```python
from build123d import *

# Parameters (mm, degrees)
PAD_DEPTH            = 10
SKETCH001_R          = 2.5
POCKET_DEPTH         = 19.79999
SKETCH002_R          = 2.125
POCKET001_DEPTH      = 28.143136
SKETCH003_R          = 4
SKETCH003_R_2        = 2.125
PAD001_DEPTH         = 5
SKETCH004_R          = 2.125
SKETCH004_R_2        = 1.5
PAD002_DEPTH         = 2
SKETCH005_W          = 20
SKETCH005_H          = 5
SKETCH005_W_2        = 9.142136
SKETCH005_H_2        = 1
POCKET002_DEPTH      = 28.143136
POCKET002_DEPTH_BACK = -10.001
SKETCH006_R          = 1.6
POCKET003_DEPTH      = 15.001
POCKET004_DEPTH      = 3
SKETCH008_R          = 5
POCKET005_DEPTH      = 2


with BuildPart() as part:
    # Sketch → Pad (new body, symmetric)
    with BuildSketch(Plane.XZ):
        Polygon((0, 0), (0, 20), (-14.142136, 34.142136), (-19.79899, 28.485281), (-8, 16.686292), (-8, 0), align=None)
    extrude(amount=PAD_DEPTH, both=True)

    # Sketch001 (on Face1 of Pad) → Pocket (cut, through all)
    with BuildSketch(Plane(origin=(0, 0, 0), x_dir=(0, 0, 1), z_dir=(1, 0, 0))):
        with Locations((10, 0)):
            Circle(SKETCH001_R)
    extrude(amount=-POCKET_DEPTH, mode=Mode.SUBTRACT)

    # Sketch002 (on Face5 of Pocket) → Pocket001 (cut, through all)
    with BuildSketch(Plane(origin=(10, 0, 10), x_dir=(-0.707107, 0, 0.707107), z_dir=(0.707107, 0, 0.707107))):
        with Locations((24.142136, 0)):
            Circle(SKETCH002_R)
    extrude(amount=-POCKET001_DEPTH, mode=Mode.SUBTRACT)

    # Sketch003 (on Face5 of Pocket001) → Pad001 (join)
    with BuildSketch(Plane(origin=(10, 0, 10), x_dir=(-0.707107, 0, 0.707107), z_dir=(0.707107, 0, 0.707107))):
        with Locations((24.142136, 0)):
            Circle(SKETCH003_R)
        with Locations((24.142136, 0)):
            Circle(SKETCH003_R_2, mode=Mode.SUBTRACT)
    extrude(amount=PAD001_DEPTH)

    # Sketch004 (on Face11 of Pad001) → Pad002 (join)
    with BuildSketch(Plane(origin=(13.535534, 0, 13.535534), x_dir=(-0.707107, 0, 0.707107), z_dir=(0.707107, 0, 0.707107))):
        with Locations((24.142136, 0)):
            Circle(SKETCH004_R)
        with Locations((24.142136, 0)):
            Circle(SKETCH004_R_2, mode=Mode.SUBTRACT)
    extrude(amount=-PAD002_DEPTH)

    # Sketch005 (on Face5 of Pad002) → Pocket002 (cut, two sides)
    with BuildSketch(Plane(origin=(10, 0, 10), x_dir=(-0.707107, 0, 0.707107), z_dir=(0.707107, 0, 0.707107))) as pocket002_sk:
        with Locations((24.142136, 7.5)):
            Rectangle(SKETCH005_W, SKETCH005_H)
        with Locations((24.142136, -7.5)):
            Rectangle(SKETCH005_W, SKETCH005_H)
        with Locations((29.571068, 0)):
            Rectangle(SKETCH005_W_2, SKETCH005_H_2)
    extrude(amount=-POCKET002_DEPTH, mode=Mode.SUBTRACT)
    extrude(pocket002_sk.sketch, amount=-POCKET002_DEPTH_BACK, mode=Mode.SUBTRACT)

    # Sketch006 (on Face16 of Pocket002) → Pocket003 (cut, through all)
    with BuildSketch(Plane.XZ.offset(5)):
        with Locations((-14.142136, 28.485281)):
            Circle(SKETCH006_R)
    extrude(amount=-POCKET003_DEPTH, mode=Mode.SUBTRACT)

    # Sketch007 (on Face10 of Pocket003) → Pocket004 (cut)
    with BuildSketch(Plane(origin=(0, 5, 0), x_dir=(1, 0, 0), z_dir=(0, 1, 0))):
        Polygon((-11.002877, -29.326443), (-11.844039, -26.187184), (-14.983298, -25.346022), (-17.281395, -27.644119), (-16.440233, -30.783378), (-13.300974, -31.62454), align=None)
    extrude(amount=-POCKET004_DEPTH, mode=Mode.SUBTRACT)

    # Sketch008 (on Face9 of Pocket004) → Pocket005 (cut)
    with BuildSketch(Plane(origin=(-8, 0, 0), x_dir=(0, 0, -1), z_dir=(-1, 0, 0))):
        with Locations((-10, 0)):
            Circle(SKETCH008_R)
    extrude(amount=-POCKET005_DEPTH, mode=Mode.SUBTRACT)


solid = part.part
```
Geometry: final body of the model. Coordinates: model frame, mm. A direction names the side the tool comes from. Coordinates: 2 decimals unless noted, no trailing zeros. Order: outer loops, then holes, each group sorted by start corner. A loop starts at its lowest first (then second) coordinate and runs counter-clockwise, first axis right, second up. Notation, with made-up numbers: (74, 62.25) -> (96, 62.25) arc R24 ccw to (96, 81.25) -> close; hole circle Ø5 at (9.5, -5.5). An arc over 180 degrees is marked (long way). Write each question's results on one line, items separated by ' | '. Start each with the question number.
1) Material intervals for line 1 along Y through (x, z) = (-6.75, 10); line 2 along Z through (x, y) = (-3.25, 1.75); line 3 along Y through (x, z) = (-16.25, 31), sorted ascending.
2) Cut plane D-D, the plane x = -13.75. State how many separate pieces and enclosed holes the cut face has, and give its area (3 significant figures).
3) Cut plane C-C, the plane z = 6. Output: boundary loops of the cut face in (x, y), and give its area (3 significant figures).
4) Mould query, pull axis X, two halves, no side actions, for faces 5 (the cylindrical face through (-7.39, -0.09, 23.75)), 6 (the flat face through (-4, -10, 8)), 7 (the flat face through (-8, -0.1, 4.8)). Classes: released by +X, released by -X, zero draft, split by the parting line, or undercut.
5) Cut plane B-B, the plane y = 0. Output: boundary loops of the cut face in (x, z).
6) Set-up query: faces 1 (the flat face through (-4, 8, 16)), 2 (the flat face through (-13.392, 3.521, 25.772)), 3 (the cylindrical face through (-7.01, -1.5, 5.23)), 4 (the flat face through (-12, -0.5, 30)). Return all of +Z, -Z, +X, -X, +Y, -Y with unobstructed straight access to the full face (end or side cutting, diameter ignored); none if empty.
7) First-contact query: pin 1 (3 mm diameter, centred on y = 0.5, z = 9, fed in from -X); pin 2 (3.5 mm diameter, centred on x = -14.14, z = 28.49, fed in from +Y); pin 3 (3 mm diameter, centred on y = 2, z = 25, fed in from +X); pin 4 (1.5 mm diameter, centred on x = -14, z = 20, fed in from +Y). Flat tips, straight axial feed; report the tip coordinate or a pass-through.
8) Cut plane A-A, the plane z = 10. Output: boundary loops of the cut face in (x, y).
Checks:
1) line 1: -10 to -5, 5 to 10 | line 2: 0 to 8.21, 11.79 to 23.25, 25.81 to 30.32 | line 3: -5 to -0.5, 0.5 to 5
2) separate pieces: 4 | enclosed holes: 0 | area: 64.6 mm^2
3) outline: (-8, -10) -> (0, -10) -> (0, 10) -> (-8, 10) -> (-8, 3) -> (-6, 3) -> (-6, -3) -> (-8, -3) -> close | area: 148 mm^2
4) face 5: undercut | face 6: zero draft | face 7: released by -X
5) outline: (-11.23, 19.91) -> (-8, 16.69) -> (-8, 15) -> (-6, 15) -> (-6, 12.5) -> (0, 12.5) -> (0, 20) -> (-4.24, 24.24) -> (-0.71, 27.78) -> (-2.47, 29.55) -> (-3.89, 28.13) -> (-3.45, 27.69) -> close; (-8, 0) -> (0, 0) -> (0, 7.5) -> (-6, 7.5) -> (-6, 5) -> (-8, 5) -> close
6) face 1: +Z, -X, +Y | face 2: +Y | face 3: -X | face 4: +Z, -X
7) pin 1: x = -6 | pin 2: y = 2 | pin 3: x = -2.47 | pin 4: through
8) outline: (-8, -10) -> (0, -10) -> (0, -2.5) -> (-6, -2.5) -> (-6, -5) -> (-8, -5) -> close; (-8, 5) -> (-6, 5) -> (-6, 2.5) -> (0, 2.5) -> (0, 10) -> (-8, 10) -> close
